Geometry: final body of the model. Coordinates: model frame, mm. A direction names the side the tool comes from. Coordinates: 2 decimals unless noted, no trailing zeros. Loops run counter-clockwise (first coordinate to the right, second up) from the corner with the lowest first, then second, coordinate; pieces in that order, holes last. Notation, with made-up numbers: (69, -2) - (75, -2) arc R10 cw to (75, 15) - close; hole circle Ø9 at (61.25, 38.25). An arc over 180 degrees is marked (long way). Return JSON: item names as keys, results as strings.
from build123d import *

# Parameters (mm, degrees)
BOSS_EXTRUDE1_DEPTH     = 16.6
BOSS_EXTRUDE2_DEPTH     = 16.6
CUT_EXTRUDE1_START      = 1.5
CUT_EXTRUDE1_DEPTH      = 13.6
CUT_EXTRUDE2_REACH      = 31.238
CUT_EXTRUDE2_END_RADIUS = 8
SKETCH3_W               = 13.6
SKETCH3_H               = 1.6
SKETCH4_W               = 13.6
SKETCH4_H               = 1.6
CUT_EXTRUDE3_DEPTH      = 1.5
FILLET1_R               = 1


with BuildPart() as part:
    # Sketch1 → Boss-Extrude1 (new body)
    with BuildSketch(Plane.XY):
        with BuildLine():
            Line((7.05, 9.5), (-7.05, 9.5))
            Line((-7.05, 9.5), (-9.903774495, 0.072462085))
            Line((-9.903774495, 0.072462085), (-7.202037804, -9.347761843))
            Line((-7.202037804, -9.347761843), (-5.760166795, -8.934230717))
            Line((-5.760166795, -8.934230717), (-7.689978717, -2.205499339))
            ThreePointArc((-7.689978717, -2.205499339), (-1.929824659, 7.763747599), (7.82763731, 1.651694325))
            Line((7.82763731, 1.651694325), (9.425731052, 1.651694325))
            Line((9.425731052, 1.651694325), (7.05, 9.5))
        make_face()
    extrude(amount=BOSS_EXTRUDE1_DEPTH)

    # Sketch2 → Boss-Extrude2 (add)
    with BuildSketch(Plane.XY):
        Polygon((-9.903774495, 0.072462085), (-7.202037804, -9.347761843), (-8.643908814, -9.761292969), (-11.467528363, 0.083903467), (-8.163157895, 11), (8.163157895, 11), (10.861396724, 2.086279273), (9.425731052, 1.651694325), (7.05, 9.5), (-7.05, 9.5), align=None)
    extrude(amount=BOSS_EXTRUDE2_DEPTH)

    # Sketch2<4> → Cut-Extrude1 (cut)
    with BuildSketch(Plane.XY.offset(CUT_EXTRUDE1_START)):
        Polygon((-9.903774495, 0.072462085), (-7.202037804, -9.347761843), (-8.643908814, -9.761292969), (-11.467528363, 0.083903467), (-8.163157895, 11), (8.163157895, 11), (10.861396724, 2.086279273), (9.425731052, 1.651694325), (7.05, 9.5), (-7.05, 9.5), align=None)
    extrude(amount=CUT_EXTRUDE1_DEPTH, mode=Mode.SUBTRACT)

    # Cut-Extrude2: up to this cylinder (the profile starts outside it)
    cut_extrude2_end = Plane(origin=(0, 0, 8.3), z_dir=(0, 0, -1)) * Cylinder(CUT_EXTRUDE2_END_RADIUS, 79.476, mode=Mode.PRIVATE)
    # Sketch3 → Cut-Extrude2 (cut, up to the surface)
    with BuildSketch(Plane(origin=(9.092549258, 2.75237134, 0), x_dir=(0, 0, -1), z_dir=(0.9571104481877781, 0.2897232989764385, 0)), mode=Mode.PRIVATE) as cut_extrude2_sk1:
        with Locations((-8.3, 1.25)):
            Rectangle(SKETCH3_W, SKETCH3_H)
    cut_extrude2_tool1 = extrude(cut_extrude2_sk1.sketch, amount=-CUT_EXTRUDE2_REACH, mode=Mode.PRIVATE) - cut_extrude2_end
    add(cut_extrude2_tool1.solids().sort_by_distance((8.730395, 3.948759, 8.3))[0], mode=Mode.SUBTRACT)

    # Sketch4 → Cut-Extrude3 (cut)
    with BuildSketch(Plane(origin=(-9.131849726, -2.619030466, 0), x_dir=(0, 0, 1), z_dir=(-0.9612473395932443, -0.2756874174221783, 0))):
        with Locations((8.3, -4.6)):
            Rectangle(SKETCH4_W, SKETCH4_H)
    extrude(amount=-CUT_EXTRUDE3_DEPTH, mode=Mode.SUBTRACT)

    # Fillet1
    fillet1_edges = [part.edges().sort_by_distance(p)[0] for p in [
        (7.82763731, 1.651694325, 8.3),
        (-5.760166795, -8.934230717, 8.3),
        (-6.725072756, -5.569865028, 16.6),
        (-1.929824659, 7.763747599, 16.6),
        (-1.929824659, 7.763747599, 0),
        (-6.725072756, -5.569865028, 0),
    ]]
    fillet(fillet1_edges, radius=FILLET1_R)


solid = part.part
Item 1: Mould query, pull axis Y, two halves, no side actions, for faces 5 (the face through (-9.838, 5.466, 0.74)), 6 (the face through (-7.426, -8.568, 8.205)), 7 (the face through (8.248, 2.967, 8.395)). Classes: +Y half, -Y half, draft (parallel to the pull), parting line (faces both ways), or undercut.
Worked out:
{"face 5": "+Y half", "face 6": "-Y half", "face 7": "undercut"}
Item 2: Ray query, probe 1 along Z at (x, y) = (7.5, 8.5); probe 2 along Y at (x, z) = (-4, 8); probe 3 along Y at (x, z) = (-2.25, 13). Return the intervals inside material, ascending. Write a range as from..to.
Worked out:
{"probe 1": "0..1.5, 15.1..16.6", "probe 2": "6.93..9.5", "probe 3": "7.68..9.5"}
Item 3: Section query A-A, the plane z = 7.5. Return loops of the section in (x, y).
Worked out:
{"outline": "(-9.9, 0.07) - (-8.08, -6.27) - (-6.64, -5.86) - (-7.69, -2.21) arc R8 cw to (6.81, 4.2) - (8.5, 4.71) - (7.05, 9.5) - (-7.05, 9.5) - close; (-7.64, -7.81) - (-7.2, -9.35) - (-6.72, -9.21) arc R1 ccw to (-6.04, -7.97) - (-6.2, -7.4) - close; (7.51, 2.74) arc R8 cw to (7.64, 2.36) arc R1 ccw to (8.6, 1.65) - (9.43, 1.65) - (8.96, 3.18) - close"}
Item 4: Reachability of faces 1 (the face through (-3, 10, 1.5)), 2 (the face through (-6.932, -7.606, 8.205)), 3 (the face through (9, 1.652, 8)), 4 (the face through (0, 9.5, 8)) from +Z, -Z, +X, -X, +Y, -Y: full face, straight path, thin tool, end or side. Return the list, or none.
Worked out:
{"face 1": "none", "face 2": "-X", "face 3": "+Z, -Z, +X, -Y", "face 4": "+X, -X, +Y"}
Item 5: First-contact query: pin 1 Ø1 at (y, z) = (1, 7) entering from +X; pin 2 Ø12 at (x, y) = (3, -4) entering from -Z; pin 3 Ø1.5 at (x, z) = (4.5, 9.5) entering from +Y; pin 4 Ø5 at (x, z) = (-7, 13) entering from -Y. Flat tips, straight axial feed; report the tip coordinate or a pass-through.
Worked out:
{"pin 1": "x = -7.86", "pin 2": "through", "pin 3": "y = 9.5", "pin 4": "y = -9.68"}
